Autodesk Inventor part; units mm, degrees
ref_plane "YZ Plane" through (0, 0, 0) normal (1, 0, 0) x (0, 1, 0)
ref_plane "XZ Plane" through (0, 0, 0) normal (0, 1, 0) x (-1, 0, 0)
ref_plane "XY Plane" through (0, 0, 0) normal (0, 0, 1) x (1, 0, 0)
sketch "Esboço1" plane through (0, 0, 0) normal (1, 0, 0) x (0, 1, 0)
  line L0 (0, 0) -> (50.8, 0)
  line L1 (50.8, 0) -> (50.8, -86.2)
  line L2 (50.8, -86.2) -> (0, -86.2)
  line L3 (0, -86.2) -> (0, 0)
  circle A0 centre (38.1, -5) radius 2.5
  circle A1 centre (25.4, -5) radius 2.5
  circle A2 centre (12.7, -5) radius 2.5
  circle A3 centre (38.1, -17.7) radius 2.5
  circle A4 centre (25.4, -17.7) radius 2.5
  circle A5 centre (12.7, -17.7) radius 2.5
  circle A6 centre (38.1, -30.4) radius 2.5
  circle A7 centre (25.4, -30.4) radius 2.5
  circle A8 centre (12.7, -30.4) radius 2.5
  circle A9 centre (38.1, -43.1) radius 2.5
  circle A10 centre (25.4, -43.1) radius 2.5
  circle A11 centre (12.7, -43.1) radius 2.5
  circle A12 centre (38.1, -55.8) radius 2.5
  circle A13 centre (25.4, -55.8) radius 2.5
  circle A14 centre (12.7, -55.8) radius 2.5
  circle A15 centre (38.1, -68.5) radius 2.5
  circle A16 centre (25.4, -68.5) radius 2.5
  circle A17 centre (12.7, -68.5) radius 2.5
  circle A18 centre (38.1, -81.2) radius 2.5
  circle A19 centre (25.4, -81.2) radius 2.5
  circle A20 centre (12.7, -81.2) radius 2.5
  dimension "d0" = 50.8
  dimension "d1" = 86.2
  dimension "d2" = 5
  dimension "d3" = 5
  dimension "d4" = 5
  dimension "d5" = 5
  dimension "d6" = 5
  dimension "d7" = 5
  dimension "d8" = 12.7
  dimension "d9" = 12.7
  dimension "d10" = 12.7
  dimension "d13" = 12.7
extrude "Extrusão1" add sketch "Esboço1" along normal blind 5
sketch "Esboço2" plane through (0, 0, 0) normal (-1, 0, 0) x (0, 0, 1)
  line L0 (-86.2, 0) -> (-149.7, 0)
  line L1 (-149.7, 0) -> (-149.7, 50.8)
  line L2 (-149.7, 50.8) -> (-86.2, 50.8)
  line L3 (-86.2, 50.8) -> (-86.2, 0)
  circle A0 centre (-144.7, 38.1) radius 2.5
  circle A1 centre (-144.7, 25.4) radius 2.5
  circle A2 centre (-144.7, 12.7) radius 2.5
  circle A3 centre (-132, 12.7) radius 2.5
  circle A4 centre (-132, 25.4) radius 2.5
  circle A5 centre (-132, 38.1) radius 2.5
  circle A6 centre (-119.3, 38.1) radius 2.5
  circle A7 centre (-119.3, 25.4) radius 2.5
  circle A8 centre (-119.3, 12.7) radius 2.5
  circle A9 centre (-106.6, 12.7) radius 2.5
  circle A10 centre (-93.9, 12.7) radius 2.5
  circle A11 centre (-93.9, 25.4) radius 2.5
  circle A12 centre (-106.6, 25.4) radius 2.5
  circle A13 centre (-106.6, 38.1) radius 2.5
  circle A14 centre (-93.9, 38.1) radius 2.5
  point P0 (0, 0)
  dimension "d20" = 50.8
  dimension "d21" = 5
extrude "Extrusão2" add sketch "Esboço2" against normal blind 5
sketch "Esboço3" plane through (0, 0, 0) normal (-1, 0, 0) x (0, 0, 1)
  circle A0 centre (-121.1, 85.9607) radius 4.5847
  circle A1 centre (63.725, 144.496) radius 17.5
  circle A2 centre (51.025, 169.896) radius 2.5
  circle A3 centre (76.425, 169.896) radius 2.5
  circle A4 centre (76.425, 119.096) radius 2.5
  circle A5 centre (51.025, 119.096) radius 2.5
  circle A6 centre (-121.1, 85.9607) radius 14.25
  circle A7 centre (63.725, 144.496) radius 20
  line L0 (-149.7, 50.8) -> (0, 50.8)
  line L1 (-149.7, 50.8) -> (-149.7, 85.9607)
  arc A8 (86.0063, 114.3333) -> (50.7735, 179.6885) centre (63.725, 144.496) ccw
  arc A9 (-130.9776, 112.8008) -> (-149.7, 85.9607) centre (-121.1, 85.9607) ccw
  line L2 (50.7735, 179.6885) -> (-130.9776, 112.8008)
  line L3 (0, 50.8) -> (0, 0)
  line L4 (0, 50.8) -> (86.0063, 114.3333)
  dimension "d26" = 28.5
  dimension "d27" = 40
  dimension "d28" = 75
extrude "Extrusão3" add sketch "Esboço3" against normal blind 5 contours L1 A9 L2 A8 L4 L0
fillet "Arredondamento1" radius 5 3 edges at (2.5, 50.8, 0) (2.5, 0, 0) (2.5, 0, -149.7)
sketch "Esboço4" plane through (0, 0, 0) normal (-1, 0, 0) x (0, 0, 1)
  line L0 (-233.5954, 270.0952) -> (45.2176, 111.8812)
  line L1 (50.7735, 179.6885) -> (-130.9776, 112.8008)
  circle A0 centre (-22.4585, 147.4099) radius 2.5
  point P0 (0, 0)
  dimension "d34" = 5
  dimension "d35" = 5
extrude "Extrusão4" cut sketch "Esboço4" against normal through all
equation "\"d6\" = d5"
equation "\"d7\" = d6"
equation "\"d9\" = d8"
equation "\"d10\" = d9"
properties part number "CHAPA FIXAÇÃO ESQUERDA 1 V2"
Input: part model. Units: mm. Frame: model coordinates. Coordinates: 2 decimals unless noted, no trailing zeros. Loops run counter-clockwise (first coordinate to the right, second up) from the corner with the lowest first, then second, coordinate; pieces in that order, holes last. Notation, with made-up numbers: M 64,63 L 74,63 A25 cw 74,78 Z; hole C -39.5,51 d5. An arc over 180 degrees is marked long. One line per item, written item: value.
(1) Section A-A (z = -81.2). Output: boundary loops of the cut face in (x, y), and give its area (3 significant figures).
Filled in:
outline: M 0,0 L 5,0 L 5,10.2 L 0,10.2 Z; M 0,15.2 L 5,15.2 L 5,22.9 L 0,22.9 Z; M 0,27.9 L 5,27.9 L 5,35.6 L 0,35.6 Z; M 0,40.6 L 5,40.6 L 5,131.12 L 0,131.12 Z
area: 581 mm^2
(2) Section C-C (z = -119.3). Output: boundary loops of the cut face in (x, y), and give its area (3 significant figures).
Filled in:
outline: M 0,0 L 5,0 L 5,10.2 L 0,10.2 Z; M 0,15.2 L 5,15.2 L 5,22.9 L 0,22.9 Z; M 0,27.9 L 5,27.9 L 5,35.6 L 0,35.6 Z; M 0,40.6 L 5,40.6 L 5,71.82 L 0,71.82 Z; M 0,100.1 L 5,100.1 L 5,117.1 L 0,117.1 Z
area: 369 mm^2
(3) Pull-direction query (Z, two-part tool) for faces 1 (the cylindrical face through (2.465, 13.451, -116.915)), 2 (the cylindrical face through (2.465, 26.151, -129.615)), 3 (the cylindrical face through (2.54, 1.43, -148.2)), 4 (the flat face through (2, 26, 0)); classes: +Z half, -Z half, draft (parallel to the pull), parting line (faces both ways), or undercut.
Filled in:
face 1: undercut
face 2: undercut
face 3: -Z half
face 4: +Z half
(4) Section D-D (x = 1.5). Give the number of separate pieces and of enclosed holes in the cut face, and give its area (3 significant figures).
Filled in:
separate pieces: 1
enclosed holes: 43
area: 25,700 mm^2
(5) Section B-B (y = 137.5). Output: boundary loops of the cut face in (x, z).
Filled in:
outline: M 0,-63.86 L 5,-63.86 L 5,44.99 L 0,44.99 Z; M 0,82.46 L 5,82.46 L 5,100.57 L 0,100.57 Z
(6) Line query: line 1 along Y through (x, z) = (2.9, 74.5); line 2 along Z through (x, y) = (3.5, 33); line 3 along Y through (x, z) = (4.6, -70). Output: solid intervals per line, ascending. Write a range as from..to.
Filled in:
line 1: 105.83..117.5, 120.69..127.65, 161.35..168.3, 171.49..180.41
line 2: -149.7..0
line 3: 0..10.7, 14.7..23.4, 27.4..36.1, 40.1..135.24
